Build history of the part. All positions in model axes, mm. A direction names the side the tool comes from. Round coordinates to 2 decimals unless told otherwise and drop trailing zeros. Write each loop counter-clockwise with the first axis right and the second up, starting at its lowest first coordinate (ties: lowest second). Pieces come first, ordered by that corner, then holes. Notation, with made-up numbers: (68.5, 29) - (103.5, 29) arc R12 cw to (103.5, 37) - close; hole circle Ø4 at (17, 19.5). An arc over 180 degrees is marked (long way). Answer as a JSON object with one key per item and string values. Group by question number.
Item 1: Probe line 1 (X direction, y = 34.5, z = 746); line 2 (Y direction, x = 257.5, z = 556.5); line 3 (Y direction, x = 126, z = 258.5). List the from-to ranges inside material, lowest first. Write a range as from..to.
Item 2: Flat gauge pins, fed straight in: pin 1 (12 mm diameter, centred on x = 182.5, z = 406.5, fed in from +Y); pin 2 (1.5 mm diameter, centred on x = 183, z = 240, fed in from +Y); pin 3 (10 mm diameter, centred on x = 75, z = 217, fed in from -Y). Where does each tip first touch, or does it go through?
Item 3: Slice it at A-A, the plane z = 710.5. List the corners of the cut face in (x, y).
Item 4: Which spindle directions (+Z, -Z, +X, -X, +Y, -Y) get a long thin tool onto all of the face, cutting with end or side? Do faces 1 (the flat face through (256, 722.608, 592)), 2 (the flat face through (1.6, 216, 592)). Say none if no direction does.
Item 5: Slice it at B-B, the plane x = 223.5. List the corners of the cut face in (y, z), then the cut area to 3 significant figures.
Item 6: Slice it at C-C, the plane y = 74. List the corners of the cut face in (x, z), then the cut area to 3 significant figures.
Autodesk Inventor part; units mm, degrees
ref_plane "YZ Plane" through (0, 0, 0) normal (1, 0, 0) x (0, 1, 0)
ref_plane "XZ Plane" through (0, 0, 0) normal (0, 1, 0) x (-1, 0, 0)
ref_plane "XY Plane" through (0, 0, 0) normal (0, 0, 1) x (1, 0, 0)
sketch "Sketch1" plane through (0, 0, 0) normal (0, 0, 1) x (1, 0, 0)
  line L0 (0, 0) -> (0, 440)
  line L1 (0, 440) -> (197.8839, 722.6075)
  line L2 (197.8839, 722.6075) -> (314.8839, 722.6075)
  dimension "d0" = 440
  dimension "d1" = 345
  dimension "d2" = 145
  dimension "d3" = 117
contour flange "Contour Flange1" sketch "Sketch1" thickness 1.6 bend radius 1.6 width 1200 along (0, 0, 1) mid plane no both sides no wall seen from (0, 220, 0) lies toward (1, 0, 0) curves L0 L1 L2
bend "Bend1"
corner "Corner1"
equation "\"d4\" = Thickness"
equation "\"d5\" = BendReliefWidth"
equation "\"d6\" = BendReliefDepth"
equation "\"d7\" = MinimumRemnant"
equation "\"d8\" = TransitionRadius"
equation "\"d10\" = BendRadius"
equation "\"d12\" = CornerReliefSize"
equation "\"d13\" = GapSize"
equation "\"d14\" = JacobiRadiusSize"
equation "\"BendRadius\" = Thickness"
equation "\"BendReliefWidth\" = Thickness"
equation "\"BendReliefDepth\" = 0.5 * Thickness"
equation "\"CornerReliefSize\" = 4 * Thickness"
equation "\"MinimumRemnant\" = 2 * Thickness"
equation "\"TransitionRadius\" = BendRadius"
equation "\"JacobiRadiusSize\" = BendRadius"
equation "\"GapSize\" = Thickness"
properties part number "Cover Front Witrh Center Point" material "Stainless Steel"
Geometry says:
{
 "1": {"line 1": "x = 0..1.6", "line 2": "y = 721.01..722.61", "line 3": "y = 617.16..619.95"},
 "2": {"pin 1": "stops at y = 709.21", "pin 2": "stops at y = 702.42", "pin 3": "stops at y = 537.18"},
 "3": {"outline": "(0, 0) - (1.6, 0) - (1.6, 438.99) arc R1.6 cw to (1.89, 439.91) - (198.24, 720.33) arc R1.6 cw to (199.55, 721.01) - (314.88, 721.01) - (314.88, 722.61) - (199.55, 722.61) arc R3.2 ccw to (196.93, 721.24) - (0.58, 440.83) arc R3.2 ccw to (0, 438.99) - close"},
 "4": {"face 1": "+Z, -Z, +X, -X, +Y", "face 2": "+Z, -Z, +X, -Y"},
 "5": {"outline": "(721.01, 0) - (722.61, 0) - (722.61, 1200) - (721.01, 1200) - close", "area": "1,920 mm^2"},
 "6": {"outline": "(0, 0) - (1.6, 0) - (1.6, 1200) - (0, 1200) - close", "area": "1,920 mm^2"}
}
